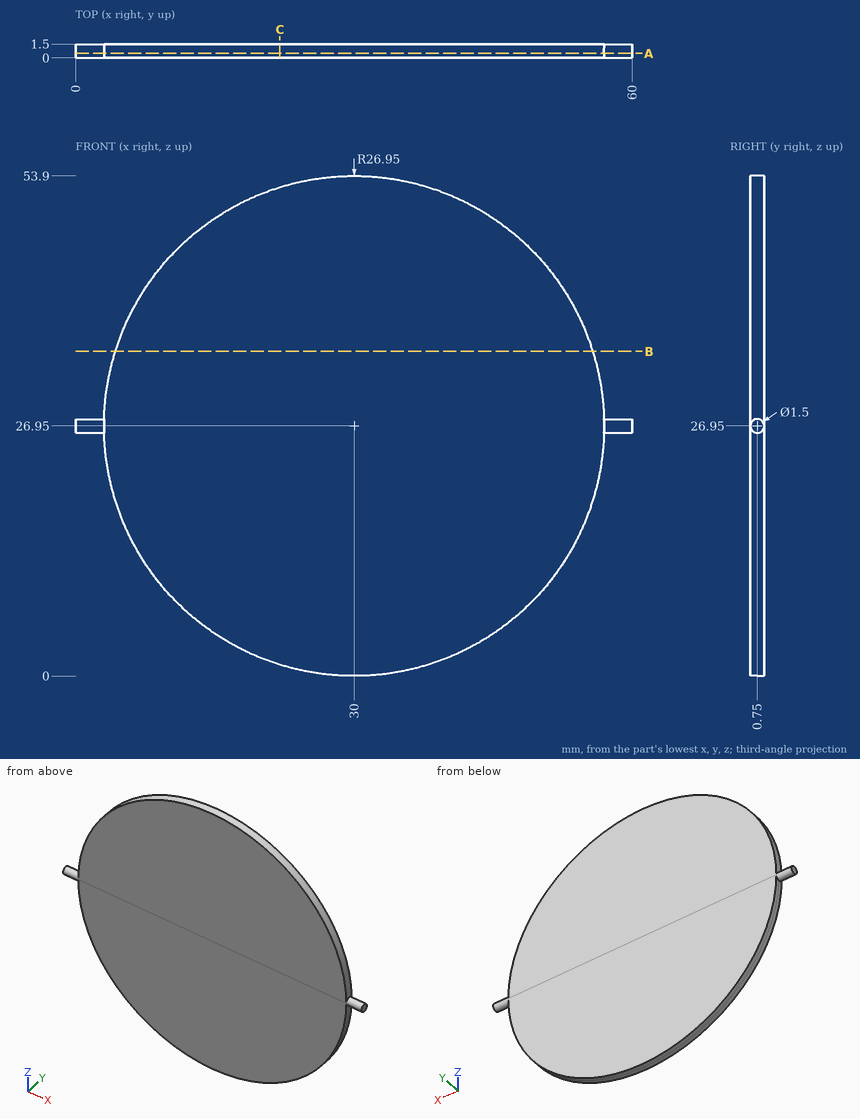
Input: dimensioned drawing with shaded views. Units: mm. Origin: part minimum x, y, z. Round coordinates to 2 decimals unless told otherwise and drop trailing zeros. Order: outer loops, then holes, each group sorted by start corner. A loop starts at its lowest first (then second) coordinate and runs counter-clockwise, first axis right, second up. Notation, with made-up numbers: (60, 42.25) -> (102, 42.25) arc R9 cw to (102, 53.25) -> close; hole circle Ø4 at (76, 4.5). An arc over 180 degrees is marked (long way). One line per item, written item: value. Start each with the question number.
Q1. Section query B-B (z = 35). Return the cut outline in (x, y), plus the area to 3 significant figures.
Q2. Section query A-A (y = 0.5). Return the cut outline in (x, z), plus the area to 3 significant figures.
Q3. Material intervals for probe 1 along Z at (x, y) = (3, 0.75); probe 2 along Z at (x, y) = (6, 1.05); probe 3 along X at (y, z) = (0.7, 38), sorted ascending.
Q4. Section query C-C (x = 22). Return the cut outline in (y, z).
Findings below:
1. outline: (4.28, 0) -> (55.72, 0) -> (55.72, 1.5) -> (4.28, 1.5) -> close
1. area: 77.2 mm²
2. outline: (0, 26.24) -> (3.06, 26.24) arc R26.95 ccw to (56.94, 26.24) -> (60, 26.24) -> (60, 27.66) -> (56.94, 27.66) arc R26.95 ccw to (3.06, 27.66) -> (0, 27.66) -> close
2. area: 2,290 mm²
3. probe 1: 26.2 to 27.7
3. probe 2: 14.69 to 39.21
3. probe 3: 5.42 to 54.58
4. outline: (0, 1.21) -> (1.5, 1.21) -> (1.5, 52.69) -> (0, 52.69) -> close
